Could you check a few things on this model? Use its own coordinates, in mm. Round coordinates to 2 decimals unless told otherwise and drop trailing zeros. Write each loop counter-clockwise with the first axis right and the second up, starting at its lowest first coordinate (ties: lowest second). Pieces come first, ordered by that corner, then holes. Notation, with made-up numbers: (18, 36) -> (34, 36) arc R22 cw to (34, 69) -> close; hole circle Ø9 at (56, 63). An arc over 180 degrees is marked (long way). Answer in a Markdown table with one row per item.
from build123d import *

# Parameters (mm, degrees)
F0_R          = 24.13
F0_R_2        = 20.447
F1_DEPTH      = 1130.3
F3_DEPTH      = 24.131
F3_DEPTH_BACK = 24.131
F5_DEPTH      = 24.131
F5_DEPTH_BACK = 24.131
F8_W          = 230.4114792496
F8_H          = 177.8236068785
F9_DEPTH      = 25.4
F9_DEPTH_BACK = 20.32


with BuildPart() as f1:
    # F0 (on Top) → F1 (new body)
    with BuildSketch(Plane.XY):
        Circle(F0_R)
        Circle(F0_R_2, mode=Mode.SUBTRACT)
    extrude(amount=F1_DEPTH)

    # F2 (on Right) → F3 (cut, two sides)
    with BuildSketch(Plane.YZ) as f3_sk:
        Polygon((24.13, 1089.8050517994), (24.13, 1130.3), (-24.13, 1130.3), align=None)
    extrude(amount=-F3_DEPTH, mode=Mode.SUBTRACT)
    extrude(f3_sk.sketch, amount=F3_DEPTH_BACK, mode=Mode.SUBTRACT)

    # F4 (on Front) → F5 (cut, two sides)
    with BuildSketch(Plane.XZ) as f5_sk:
        Polygon((-28.575, 0), (28.575, 0), (28.575, 26.6494826636), align=None)
    extrude(amount=F5_DEPTH, mode=Mode.SUBTRACT)
    extrude(f5_sk.sketch, amount=-F5_DEPTH_BACK, mode=Mode.SUBTRACT)

    # F8 (on line) → F9 (cut, two sides)
    with BuildSketch(Plane(origin=(-2.5518360133, -6.0381584146, 5.4724299905), x_dir=(-0.9543044076, 0.2214273865, -0.2006813646), z_dir=(0.2988362387, 0.7071067812, -0.6408563821))) as f9_sk:
        with Locations((9.1961668804, 17.1195510775)):
            Rectangle(F8_W, F8_H)
    extrude(amount=F9_DEPTH, mode=Mode.SUBTRACT)
    extrude(f9_sk.sketch, amount=-F9_DEPTH_BACK, mode=Mode.SUBTRACT)


solid = f1.part
1) For pin 1 (5 mm diameter, centred on x = 18, z = 737, fed in from +Y); pin 2 (10 mm diameter, centred on y = -9.5, z = 816.5, fed in from +X); pin 3 (4 mm diameter, centred on y = 17, z = 588.5, fed in from -X), each with a flat end and sliding along its axis, tell me the tip position at first contact or that it passes through.
Findings:
| item | result |
|---|---|
| pin 1 | stops at y = 18.49 |
| pin 2 | stops at x = 23.71 |
| pin 3 | stops at x = -18.9 |
2) Imagine slicing it at B-B, the plane x = -9. Please give me the cut outline in (y, z), plus the area to 3 significant figures.
Findings:
| item | result |
|---|---|
| outline | (-22.39, 16.13) -> (-18.36, 20.58) -> (-18.36, 1125.46) -> (-22.39, 1128.84) -> close; (18.36, 61.09) -> (22.39, 65.54) -> (22.39, 1091.27) -> (18.36, 1094.65) -> close |
| area | 8,620 mm^2 |
3) Imagine slicing it at A-A, the plane y = 0. Please give me the cut outline in (x, z).
Findings:
| item | result |
|---|---|
| outline | (-24.13, 33.78) -> (-20.45, 35.5) -> (-20.45, 1110.05) -> (-24.13, 1110.05) -> close; (20.45, 54.57) -> (24.13, 56.28) -> (24.13, 1110.05) -> (20.45, 1110.05) -> close |
4) Imagine slicing it at C-C, the plane z = 840.5. Please give me the cut outline in (x, y).
Findings:
| item | result |
|---|---|
| outline | circle Ø48.26 at (0, 0); hole circle Ø40.89 at (0, 0) |
5) Thinking about a two-plate mould opening in Y: for faces 1 (the face through (-21.561, -0.113, 1110.147)), 2 (the face through (-16.226, -12.442, 565.846)), 3 (the face through (-5.231, -23.556, 565.203)), which applies, +Y half, -Y half, draft (parallel to the pull), parting line (faces both ways), or undercut?
Findings:
| item | result |
|---|---|
| face 1 | +Y half |
| face 2 | undercut |
| face 3 | parting line |
6) Please list where these lines run through material, in increasing order: line 1 (Y direction, x = -1.5, z = 936.5); line 2 (X direction, y = 0, z = 499); line 3 (X direction, y = -3, z = 768).
Findings:
| item | result |
|---|---|
| line 1 | y = -24.08 to -20.39, 20.39 to 24.08 |
| line 2 | x = -24.13 to -20.45, 20.45 to 24.13 |
| line 3 | x = -23.94 to -20.23, 20.23 to 23.94 |
